Source: CAD feature listing. Evaluate the final solid. Frame: model axes, mm. A direction names the side the tool comes from. Round coordinates to 2 decimals unless told otherwise and drop trailing zeros. Loops run counter-clockwise (first coordinate to the right, second up) from the corner with the lowest first, then second, coordinate; pieces in that order, holes last. Notation, with made-up numbers: (20.25, 84) - (48.25, 84) arc R24 ccw to (48.25, 114) - close; hole circle Ø5 at (21, 42.25). An arc over 180 degrees is marked (long way). One line per question, with ' | ' between items.
from build123d import *

# Parameters (mm, degrees)
BOSS_EXTRUDE1_DEPTH = 5


with BuildPart() as part:
    # Sketch1 → Boss-Extrude1 (new body)
    with BuildSketch(Plane(origin=(0, 0, 0), x_dir=(1, 0, 0), z_dir=(0, 1, 0))):
        with BuildLine():
            Line((0, -2), (8, -2))
            ThreePointArc((8, -2), (9.414213562, -1.414213562), (10, 0))
            Line((10, 0), (10, 23))
            ThreePointArc((10, 23), (10.585786438, 24.414213562), (12, 25))
            Line((12, 25), (45, 25))
            ThreePointArc((45, 25), (46.414213562, 25.585786438), (47, 27))
            Line((47, 27), (47, 35))
            ThreePointArc((47, 35), (46.414213562, 36.414213562), (45, 37))
            Line((45, 37), (0, 37))
            ThreePointArc((0, 37), (-1.414213562, 36.414213562), (-2, 35))
            Line((-2, 35), (-2, 0))
            ThreePointArc((-2, 0), (-1.414213562, -1.414213562), (0, -2))
        make_face()
        with BuildLine():
            Line((42, 29.4), (4, 29.4))
            ThreePointArc((4, 29.4), (2.4, 31), (4, 32.6))
            Line((4, 32.6), (42, 32.6))
            ThreePointArc((42, 32.6), (43.6, 31), (42, 29.4))
        make_face(mode=Mode.SUBTRACT)
        with BuildLine():
            Line((2.4, 3), (2.4, 21))
            ThreePointArc((2.4, 21), (4, 22.6), (5.6, 21))
            Line((5.6, 21), (5.6, 3))
            ThreePointArc((5.6, 3), (4, 1.4), (2.4, 3))
        make_face(mode=Mode.SUBTRACT)
    extrude(amount=BOSS_EXTRUDE1_DEPTH)


solid = part.part
1. Mould query, pull axis Z, two halves, no side actions, for faces 4 (the flat face through (10, 2, -11)), 5 (the cylindrical face through (9.4, 2.46, 1.43)), 6 (the flat face through (5.6, 2, -12)), 7 (the flat face through (2.4, 2, -12)). Classes: released by +Z, released by -Z, zero draft, split by the parting line, or undercut.
Worked out:
face 4: zero draft | face 5: released by +Z | face 6: undercut | face 7: undercut
2. Access query for faces 1 (the flat face through (28, 2, -25)), 2 (the flat face through (17, 0, -26)), 3 (the flat face through (23, 2, -29.4)). Directions: +Z, -Z, +X, -X, +Y, -Y. A direction counts if a zero-diameter tool reaches every point of the face in a straight line with its end or side. Return the directions, or none.
Worked out:
face 1: +Z, +X, +Y, -Y | face 2: +Z, -Z, +X, -X, -Y | face 3: +Y, -Y
3. Contact query for flat-ended pins moving along their axis: P1, Ø12, axis at x = 29.5, z = -31.5, coming from the +Y side; P2, Ø1.5, axis at x = 21, y = 2, coming from the +Z side; P3, Ø2.5, axis at y = 1.5, z = -8, coming from the +X side. Output: stop coordinate, or through.
Worked out:
P1: stops at y = 5 | P2: stops at z = -25 | P3: stops at x = 10
4. Section query D-D, the plane z = -24. Return loops of the section in (x, y).
Worked out:
outline: (-2, 0) - (10.27, 0) - (10.27, 5) - (-2, 5) - close
5. Material intervals for probe 1 along Z at (x, y) = (30.5, 4.05); probe 2 along X at (y, z) = (2.3, -18); probe 3 along Z at (x, y) = (10.5, 2.9), sorted ascending.
Worked out:
probe 1: z = -37 to -32.6, -29.4 to -25 | probe 2: x = -2 to 2.4, 5.6 to 10 | probe 3: z = -37 to -32.6, -29.4 to -24.32
6. Section query B-B, the plane x = 14. Return loops of the section in (y, z).
Worked out:
outline: (0, -37) - (5, -37) - (5, -32.6) - (0, -32.6) - close; (0, -29.4) - (5, -29.4) - (5, -25) - (0, -25) - close
7. Section query C-C, the plane y = 3.65. Return loops of the section in (x, z), plus the area to 3 significant figures.
Worked out:
outline: (-2, -35) arc R2 ccw to (0, -37) - (45, -37) arc R2 ccw to (47, -35) - (47, -27) arc R2 ccw to (45, -25) - (12, -25) arc R2 cw to (10, -23) - (10, 0) arc R2 ccw to (8, 2) - (0, 2) arc R2 ccw to (-2, 0) - close; hole (2.4, -21) arc R1.6 ccw to (5.6, -21) - (5.6, -3) arc R1.6 ccw to (2.4, -3) - close; hole (4, -32.6) - (42, -32.6) arc R1.6 ccw to (42, -29.4) - (4, -29.4) arc R1.6 ccw to start | area: 713 mm2
8. Section query A-A, the plane z = -8. Return loops of the section in (x, y).
Worked out:
outline: (-2, 0) - (2.4, 0) - (2.4, 5) - (-2, 5) - close; (5.6, 0) - (10, 0) - (10, 5) - (5.6, 5) - close
